from build123d import *

# Parameters (mm, degrees)
SALIENTE_EXTRUIR1_DEPTH = 15
CROQUIS2_R              = 2.5
CORTAR_EXTRUIR2_DEPTH   = 30
CHAFL_N1_SIZE           = 5


with BuildPart() as part:
    # Croquis1 → Saliente-Extruir1 (new, symmetric)
    with BuildSketch(Plane(origin=(0, 0, 0), x_dir=(1, 0, 0), z_dir=(0, 1, 0))):
        Polygon((0, 0), (0, 186), (4, 186), (4, 4), (9, 4), (9, -14), (4, -14), (4, -64), (0, -64), (0, -10), (5, -10), (5, 0), align=None)
    extrude(amount=SALIENTE_EXTRUIR1_DEPTH, both=True)

    # Croquis2 → Cortar-Extruir2 (cut)
    with BuildSketch(Plane(origin=(0, 0, 0), x_dir=(0, 0, -1), z_dir=(1, 0, 0))):
        with Locations(Location((-51.5, 0, 0), (0, 0, 180))):
            Circle(CROQUIS2_R)
        with Locations(Location((25, 0, 0), (0, 0, 180))):
            Circle(CROQUIS2_R)
        with Locations(Location((97, 0, 0), (0, 0, 180))):
            Circle(CROQUIS2_R)
        with Locations(Location((173.5, 0, 0), (0, 0, 180))):
            Circle(CROQUIS2_R)
    extrude(amount=CORTAR_EXTRUIR2_DEPTH, mode=Mode.SUBTRACT)

    # Chaflán1
    chafl_n1_edges = [part.edges().sort_by_distance(p)[0] for p in [
        (2, -15, -186),
        (2, 15, -186),
        (2, -15, 64),
        (2, 15, 64),
        (4, 0, -4),
        (4, 0, 14),
    ]]
    chamfer(chafl_n1_edges, length=CHAFL_N1_SIZE - 0.0001)  # a hair under: the kernel refuses the full size


solid = part.part
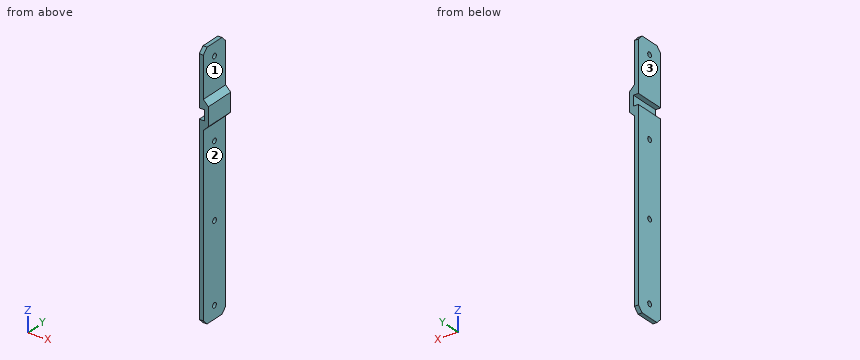
For this review, take the finished solid that the model builds, in its own axes (mm). Face numbers are marked on the shaded views. A direction names the side the tool comes from. Give positions to 0.01 mm unless a question says otherwise; leave off trailing zeros. Loops run counter-clockwise (first coordinate to the right, second up) from the corner with the lowest first, then second, coordinate; pieces in that order, holes last.
Item 1: Tool access review of the marked faces 1, 2 and 3: name each direction out of +Z, -Z, +X, -X, +Y, -Y from which nothing blocks a thin tool from reaching the whole face with its end or side.
Item 2: Take a section at B-B, the plane y = 0. Give the number of separate pieces and of enclosed holes in the cut face, and give its area (3 significant figures).
Item 3: Insertion check: pin 1 (4.5 mm diameter, centred on y = 0, z = -173.5, fed in from -X); pin 2 (5 mm diameter, centred on x = 7.5, y = -1.5, fed in from -Z); pin 3 (5 mm diameter, centred on y = 0, z = 7, fed in from -X); pin 4 (15 mm diameter, centred on y = 4, z = 31, fed in from +X). Each pin has a flat end and moves straight along its axis. Give the tip position at first contact, or say it passes through.
Item 4: Take a section at A-A, the plane z = -25. State the section outline as (x, y) points, and give its area (3 significant figures).
Item 5: For line 1 along Z through (x, y) = (2.5, -4.25); line 2 along Y through (x, z) = (2.2, -25); line 3 along X through (y, z) = (8.5, -151), list the stretches that pass through material, from the lowest coordinate up.
Item 6: Take a section at C-C, the plane z = -50.5. State the section outline as (x, y) points.
Calculated:
1. face 1: +Z, +X, +Y, -Y
1. face 2: -Z, +X, +Y, -Y
1. face 3: +Z, -Z, -X, +Y, -Y
2. separate pieces: 5
2. enclosed holes: 0
2. area: 985 mm2
3. pin 1: passes through
3. pin 2: stops at z = -8
3. pin 3: stops at x = 5
3. pin 4: stops at x = 4
4. outline: (0, -15) - (4, -15) - (4, -2.5) - (0, -2.5) - close; (0, 2.5) - (4, 2.5) - (4, 15) - (0, 15) - close
4. area: 100 mm2
5. line 1: z = -186 to 0, 10 to 64
5. line 2: y = -15 to -2.5, 2.5 to 15
5. line 3: x = 0 to 4
6. outline: (0, -15) - (4, -15) - (4, 15) - (0, 15) - close
